CAD build for the part. Positions are in the model's coordinates, mm. Face numbers are marked on the shaded views. A direction names the side the tool comes from. Coordinates: 2 decimals unless noted, no trailing zeros. Loops run counter-clockwise (first coordinate to the right, second up) from the corner with the lowest first, then second, coordinate; pieces in that order, holes last. Notation, with made-up numbers: M 64.5,-7 L 81.5,-7 A21 ccw 81.5,5 Z; hole C -9,89 d5. An arc over 180 degrees is marked long. Answer as a JSON object with one key per item and string values. Group by question number.
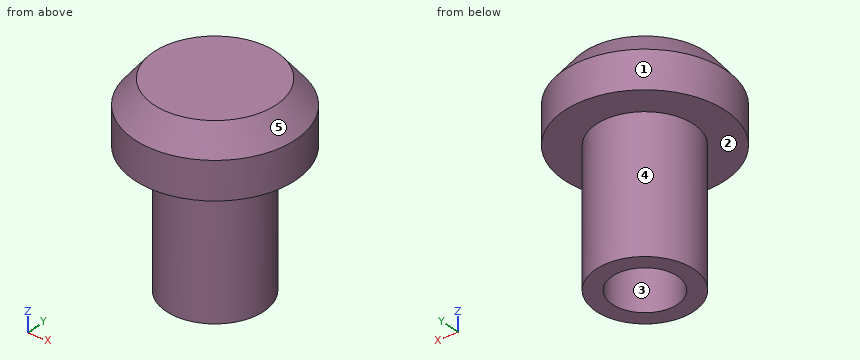
```python
from build123d import *


with BuildPart() as f1:
    # F0 (on Right) → F1 (revolve)
    with BuildSketch(Plane.YZ):
        with BuildLine():
            Line((-19.05, 0), (-12.7, 0))
            Line((-12.7, 0), (-12.7, 48.895))
            ThreePointArc((-12.7, 48.895), (-8.980256, 57.875256), (0, 61.595))
            Line((0, 61.595), (0, 76.2))
            Line((0, 76.2), (-23.871235, 76.2))
            Line((-23.871235, 76.2), (-31.409519, 66.675))
            Line((-31.409519, 66.675), (-31.409519, 52.07))
            Line((-31.409519, 52.07), (-19.05, 52.07))
            Line((-19.05, 52.07), (-19.05, 0))
        make_face()
    revolve(axis=Axis((0, 0, 68.8975), (0, 0, -1)))


solid = f1.part
```
Item 1: Pin check, flat tips, straight feed: pin 1 (5 mm diameter, centred on x = -6, z = 32.5, fed in from -Y); pin 2 (8 mm diameter, centred on x = 10, z = 9.5, fed in from -Y); pin 3 (5 mm diameter, centred on y = 18, z = 13.5, fed in from -X). Stop position of each tip, or through.
Item 2: Pull direction X, two halves, no side cores. Call the marked faces 1, 2 and 3: released by +X, released by -X, zero draft, split by the parting line, or undercut.
Item 3: Drill centre lines: L1, parallel to Y at x = 0, z = 26; L2, parallel to Z at x = -9, y = -19.5. Where is each one in solid material? Low to high. Write a range as from..to.
Item 4: Slice it at A-A, the plane z = 12. Write the cut outline in (x, y), then the cut area to 3 significant figures.
Item 5: Tool access for the marked faces 4 and 5: list every direction of +Z, -Z, +X, -X, +Y, -Y with a clear straight run to the whole face (end or side of a thin tool).
Computed:
{
 "1": {"pin 1": "y = -18.73", "pin 2": "y = -18.08", "pin 3": "x = -11.07"},
 "2": {"face 1": "split by the parting line", "face 2": "zero draft", "face 3": "undercut"},
 "3": {"L1": "-19.05..-12.7, 12.7..19.05", "L2": "52.07..76.2"},
 "4": {"outline": "C 0,0 d38.1; hole C 0,0 d25.4", "area": "633 mm2"},
 "5": {"face 4": "-Z", "face 5": "+Z"}
}
